Autodesk Inventor part; units mm, degrees
ref_plane "YZ Plane" through (0, 0, 0) normal (1, 0, 0) x (0, 1, 0)
ref_plane "XZ Plane" through (0, 0, 0) normal (0, 1, 0) x (-1, 0, 0)
ref_plane "XY Plane" through (0, 0, 0) normal (0, 0, 1) x (1, 0, 0)
sketch "Skizze2" plane through (0, 0, 0) normal (0, 1, 0) x (-1, 0, 0)
  line L0 (-6.5, 9.5) -> (6.5, 9.5)
  line L1 (6.5, 9.5) -> (6.5, -9.5)
  line L2 (6.5, -9.5) -> (-6.5, -9.5)
  line L3 (-6.5, -9.5) -> (-6.5, 9.5)
  line L4 (-6.5, 9.5) -> (6.5, -9.5) construction
  line L5 (6.5, 9.5) -> (-6.5, -9.5) construction
  point P0 (0, 0)
  dimension "d1" = 19
  dimension "d2" = 13
extrude "Extrusion1" add sketch "Skizze2" along normal blind 6
sketch "Skizze3" plane through (0, 6, 0) normal (0, 1, 0) x (1, 0, 0)
  point P0 (0, 0)
  point P1 (0, 0)
hole "Bohrung1" at (0, 6, 0) direction (0, -1, 0) diameter 6.5 depth 6
sketch "Skizze4" plane through (-6.5, 0, -9.5) normal (-1, 0, 0) x (0, 0, 1)
  circle A0 centre (9.5, 3) radius 2.5
  line L0 (0, 0) -> (0, 6)
  line L1 (0, 0) -> (19, 0)
  point P0 (9.5, 0)
  point P1 (0, 3)
  point P2 (9.5, 0)
  dimension "d12" = 5
extrude "Extrusion2" add sketch "Skizze4" along normal blind 34
sketch "Skizze5" plane through (-40.5, 3, 0) normal (-1, 0, 0) x (0, 0, 1)
  circle A0 centre (0, 0) radius 2.5
  point P0 (0, -3)
hole "Bohrung2" at (-40.5, 3, 0) direction (1, 0, 0) diameter 3.242 depth 5
properties part number "pleuel_m4"
Here's how the part is built. I have some questions about the finished solid (model axes, mm). A direction names the side the tool comes from. Coordinates: 2 decimals unless noted, no trailing zeros. Order: outer loops, then holes, each group sorted by start corner. A loop starts at its lowest first (then second) coordinate and runs counter-clockwise, first axis right, second up. Notation, with made-up numbers: (45, 83.25) - (102, 83.25) arc R20 ccw to (102, 102.25) - close; hole circle Ø1 at (-19, 5.25). An arc over 180 degrees is marked (long way). One line per question, with ' | ' between items. Start each with the question number.
1. If we mould it in two halves opening along Z, with no side actions, what happens to faces 3 (the flat face through (0, 3, 9.5)), 4 (the cylindrical face through (1.978, 2.958, -2.579)), 5 (the flat face through (6.5, 3, 0)), 6 (the flat face through (0, 3, -9.5))? For each: released by +Z, released by -Z, zero draft, split by the parting line, or undercut.
2. I'm going to push flat-ended pins straight in: pin 1 Ø1 at (x, y) = (-23, 4) entering from +Z; pin 2 Ø1.6 at (y, z) = (2.5, -0.5) entering from -X; pin 3 Ø2 at (x, y) = (-13, 2.5) entering from -Z. Where does each tip first touch, or does it pass through?
3. If we section it at D-D (x = -10.5): Write out the boundary of the cut face in (y, z), and give its area (3 significant figures).
4. If we section it at C-C (y = 3): Write out the boundary of the cut face in (x, z).
5. Please list where these lines run through material, in increasing order: line 1 along X through (y, z) = (3.35, 0); line 2 along X through (y, z) = (5, 0.25); line 3 along Y through (x, z) = (-39.35, 0). Write a range as [from, to].
6. Which directions (+Z, -Z, +X, -X, +Y, -Y) give clear straight access to the entire face, cutting with the end or side of a thin tool? Please do faces 1 (the cylindrical face through (-23.3, 4.5, -2)), 2 (the flat face through (3, 0, 2)).
7. If we section it at A-A (x = 0): Write out the boundary of the cut face in (y, z).
8. If we section it at B-B (z = 0): Write out the boundary of the cut face in (x, y), and give its area (3 significant figures).
Model answer:
1) face 3: released by +Z | face 4: undercut | face 5: zero draft | face 6: released by -Z
2) pin 1: stops at z = 2.45 | pin 2: stops at x = -35.5 | pin 3: stops at z = -2.5
3) outline: circle Ø5 at (3, 0) | area: 19.6 mm²
4) outline: (-40.5, -2.5) - (-6.5, -2.5) - (-6.5, -9.5) - (6.5, -9.5) - (6.5, 9.5) - (-6.5, 9.5) - (-6.5, 2.5) - (-40.5, 2.5) - (-40.5, 1.62) - (-35.5, 1.62) - (-35.5, -1.62) - (-40.5, -1.62) - close; hole circle Ø6.5 at (0, 0)
5) line 1: x = [-35.5, -3.25], [3.25, 6.5] | line 2: x = [-40.5, -3.24], [3.24, 6.5] | line 3: y = [0.5, 1.38], [4.62, 5.5]
6) face 1: -X | face 2: +Z, -Z, +X, -X, -Y
7) outline: (0, -9.5) - (6, -9.5) - (6, -3.25) - (0, -3.25) - close; (0, 3.25) - (6, 3.25) - (6, 9.5) - (0, 9.5) - close
8) outline: (-40.5, 0.5) - (-6.5, 0.5) - (-6.5, 0) - (-3.25, 0) - (-3.25, 6) - (-6.5, 6) - (-6.5, 5.5) - (-40.5, 5.5) - (-40.5, 4.62) - (-35.5, 4.62) - (-35.5, 1.38) - (-40.5, 1.38) - close; (3.25, 0) - (6.5, 0) - (6.5, 6) - (3.25, 6) - close | area: 193 mm²
